For this review, take the finished solid that the model builds, in its own axes (mm). Face numbers are marked on the shaded views. Round coordinates to 2 decimals unless told otherwise and drop trailing zeros. Write each loop counter-clockwise with the first axis right and the second up, starting at its lowest first coordinate (ties: lowest second). Pieces come first, ordered by that corner, then holes. Notation, with made-up numbers: (40.25, 57.5) -> (86.25, 57.5) arc R13 cw to (86.25, 78.5) -> close; hole circle Ø5 at (61.25, 39.25). An arc over 180 degrees is marked (long way). Answer in a Markdown table with one row per item.
from build123d import *

# Parameters (mm, degrees)
SKETCH3_W                = 63.5
SKETCH3_H                = 63.5
BOSS_EXTRUDE2_DEPTH      = 25.4
BOSS_EXTRUDE2_DEPTH_BACK = 25.4


with BuildPart() as part:
    # Sketch1 → Revolve1 (revolve)
    with BuildSketch(Plane.XY):
        with BuildLine():
            Line((-76.123658673, 5.804761032), (-63.20203376, 4.819430767))
            ThreePointArc((-63.20203376, 4.819430767), (-48.098438833, -41.28273448), (-4.819430767, -63.20203376))
            Line((-4.819430767, -63.20203376), (-5.804761032, -76.123658673))
            ThreePointArc((-5.804761032, -76.123658673), (-57.932141145, -49.722969368), (-76.123658673, 5.804761032))
        make_face()
    revolve(axis=Axis((0, 0, 0), (-0.076033625, -0.997105254, 0)))

    # Sketch3 → Boss-Extrude2 (add, two sides)
    with BuildSketch(Plane(origin=(-5.804761032, -76.123658673, 0), x_dir=(-0.997105254, 0.076033625, 0), z_dir=(-0.076033625, -0.997105254, 0))) as boss_extrude2_sk:
        Rectangle(SKETCH3_W, SKETCH3_H)
    extrude(amount=BOSS_EXTRUDE2_DEPTH)
    extrude(boss_extrude2_sk.sketch, amount=-BOSS_EXTRUDE2_DEPTH_BACK)


solid = part.part
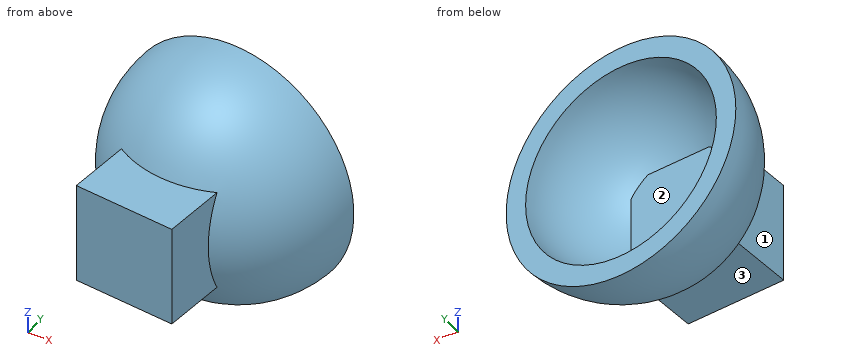
1) Consider section A-A on z = -11. State the section outline as (x, y) points, then the cut area to 3 significant figures.
Solved:
| item | result |
|---|---|
| outline | (-75.33, 5.74) arc R75.55 ccw to (-36.87, -65.94) -> (-39.39, -99.04) -> (23.92, -103.86) -> (26.45, -70.77) arc R75.55 ccw to (75.33, -5.74) -> (62.24, -4.75) arc R62.42 cw to (27.57, -56) -> (27.78, -53.21) -> (-35.53, -48.38) -> (-35.74, -51.18) arc R62.42 cw to (-62.24, 4.75) -> close |
| area | 5,200 mm² |
2) Mouldability with a two-part tool opening along Z and no side actions: class the marked faces 1, 2 and 3 as pulls with the +Z half, pulls with the -Z half, needs draft (parallel to the pull), parting line crosses it, or undercut.
Solved:
| item | result |
|---|---|
| face 1 | needs draft |
| face 2 | undercut |
| face 3 | pulls with the -Z half |
3) For line 1 (Z direction, x = 35.5, y = -28); line 2 (Z direction, x = 24, y = -34); line 3 (Z direction, x = 24, y = -83), list the stretches that pass through material, from the lowest coordinate up. Write a range as [from, to].
Solved:
| item | result |
|---|---|
| line 1 | [-61.52, -44.42], [44.42, 61.52] |
| line 2 | [-64, -47.81], [47.81, 64] |
| line 3 | [-31.75, 31.75] |
4) Consider section B-B on y = -69. State the section outline as (x, z) points.
Solved:
| item | result |
|---|---|
| outline | (-37.1, -31.75) -> (-7.71, -31.75) arc R32.67 ccw to (7.71, -31.75) -> (26.58, -31.75) -> (26.58, -19) arc R32.67 ccw to (26.58, 19) -> (26.58, 31.75) -> (7.71, 31.75) arc R32.67 ccw to (-7.71, 31.75) -> (-37.1, 31.75) -> close |
5) Consider section C-C on x = -16.5. State the section outline as (y, z) points.
Solved:
| item | result |
|---|---|
| outline | (-100.78, -31.75) -> (-67.44, -31.75) arc R74.54 ccw to (1.26, -74.53) -> (1.26, -61.19) arc R61.2 cw to (-52.32, -31.75) -> (-49.83, -31.75) -> (-49.83, 31.75) -> (-52.32, 31.75) arc R61.2 cw to (1.26, 61.19) -> (1.26, 74.53) arc R74.54 ccw to (-67.44, 31.75) -> (-100.78, 31.75) -> close |
6) Clearance check with flat-ended pins moving along their axes: pin 1 Ø10 at (x, y) = (-36, -64.5) entering from -Z; pin 2 Ø3 at (x, z) = (-21, -40) entering from -Y; pin 3 Ø8 at (x, y) = (12, -74.5) entering from -Z. State where each tip first meets the part, or that it passes through.
Solved:
| item | result |
|---|---|
| pin 1 | z = -32.95 |
| pin 2 | y = -62.62 |
| pin 3 | z = -31.75 |
7) Consider section D-D on y = -13. State the section outline as (x, z) points, then the cut area to 3 significant figures.
Solved:
| item | result |
|---|---|
| outline | circle Ø150.46 at (0, 0); hole circle Ø124.08 at (0, 0) |
| area | 5,690 mm² |
